from build123d import *

# Parameters (mm, degrees)
SKETCH_1_W          = 146
SKETCH_1_H          = 98
EXTRUDE_1_DEPTH     = 18
SKETCH_2_W          = 141
SKETCH_2_H          = 90
CUT_EXTRUDE_1_DEPTH = 14
SKETCH_3_W          = 91
SKETCH_3_H          = 90
CUT_EXTRUDE_2_DEPTH = 17
CUT_EXTRUDE_3_DEPTH = 17


with BuildPart() as part:
    # 草图1 → 凸台-拉伸1 (new body)
    with BuildSketch(Plane(origin=(0, 0, 0), x_dir=(1, 0, 0), z_dir=(0, 1, 0))):
        with Locations((-12.96875, -2.625)):
            Rectangle(SKETCH_1_W, SKETCH_1_H)
    extrude(amount=EXTRUDE_1_DEPTH)

    # 草图2 → 切除-拉伸1 (cut)
    with BuildSketch(Plane(origin=(0, 18, 0), x_dir=(1, 0, 0), z_dir=(0, 1, 0))):
        with Locations((-15.46875, -2.625)):
            Rectangle(SKETCH_2_W, SKETCH_2_H)
    extrude(amount=-CUT_EXTRUDE_1_DEPTH, mode=Mode.SUBTRACT)

    # 草图3 → 切除-拉伸2 (cut)
    with BuildSketch(Plane(origin=(0, 4, 0), x_dir=(1, 0, 0), z_dir=(0, 1, 0))):
        with Locations((9.53125, -2.625)):
            Rectangle(SKETCH_3_W, SKETCH_3_H)
    extrude(amount=-CUT_EXTRUDE_2_DEPTH, mode=Mode.SUBTRACT)

    # 草图5 → 切除-拉伸3 (cut)
    with BuildSketch(Plane(origin=(0, 4, 0), x_dir=(1, 0, 0), z_dir=(0, 1, 0))):
        with BuildLine():
            Line((-73.931388989, 24.875), (-77.931388989, 24.875))
            ThreePointArc((-77.931388989, 24.875), (-79.431388989, 26.375), (-77.931388989, 27.875))
            Line((-77.931388989, 27.875), (-73.931388989, 27.875))
            ThreePointArc((-73.931388989, 27.875), (-72.431388989, 26.375), (-73.931388989, 24.875))
        make_face()
        with BuildLine():
            Line((-73.931388989, 7.375), (-77.931388989, 7.375))
            ThreePointArc((-77.931388989, 7.375), (-79.431388989, 8.875), (-77.931388989, 10.375))
            Line((-77.931388989, 10.375), (-73.931388989, 10.375))
            ThreePointArc((-73.931388989, 10.375), (-72.431388989, 8.875), (-73.931388989, 7.375))
        make_face()
    extrude(amount=-CUT_EXTRUDE_3_DEPTH, mode=Mode.SUBTRACT)


solid = part.part
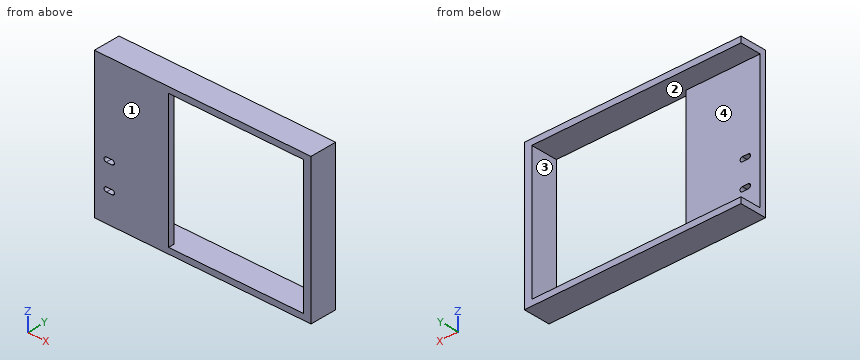
Input: part model. Units: mm. Frame: model coordinates. Face numbers are marked on the shaded views. A direction names the side the tool comes from. Give positions to 0.01 mm unless a question says otherwise; leave off trailing zeros. Write each loop counter-clockwise with the first axis right and the second up, starting at its lowest first coordinate (ties: lowest second). Pieces come first, ordered by that corner, then holes.
Q1. Section D-D, the plane x = -52. Output: boundary loops of the cut face in (y, z) (3 decimals), plus the area to 3 significant figures.
Q2. Material intervals for probe 1 along Z at (x, y) = (-60, 11.5) (3 decimals); probe 2 along X at (y, z) = (2.5, 43); probe 3 along X at (y, z) = (5.5, 30), sorted ascending.
Q3. Set-up query: the marked faces 1, 2, 3 and 4. Return all of +Z, -Z, +X, -X, +Y, -Y with unobstructed straight access to the full face (end or side cutting, diameter ignored); none if empty.
Q4. Section C-C, the plane y = 2. Output: boundary loops of the cut face in (x, z) (3 decimals), plus the area to 3 significant figures.
Q5. First-contact query: P1, Ø6, axis at x = -38.5, z = 30, coming from the +Y side. Flat tip, straight axial feed; report the tip coordinate or a pass-through.
Q6. Section B-B, the plane z = 0. Output: boundary loops of the cut face in (x, y), plus the area to 3 significant figures.
Q7. Section A-A, the plane x = -1. Output: boundary loops of the cut face in (y, z) (3 decimals), plus the area to 3 significant figures.
Filled in:
1. outline: (0, -46.375) - (18, -46.375) - (18, -42.375) - (4, -42.375) - (4, 47.625) - (18, 47.625) - (18, 51.625) - (0, 51.625) - close
1. area: 504 mm2
2. probe 1: z = -46.375 to -42.375, 47.625 to 51.625
2. probe 2: x = -85.97 to -35.97, 55.03 to 60.03
2. probe 3: x = 55.03 to 60.03
3. face 1: +Z, -Z, +X, -X, -Y
3. face 2: +Y
3. face 3: +Y, -Y
3. face 4: -X, +Y
4. outline: (-85.969, -46.375) - (60.031, -46.375) - (60.031, 51.625) - (-85.969, 51.625) - close; hole (-77.931, -27.875) - (-73.931, -27.875) arc R1.5 ccw to (-73.931, -24.875) - (-77.931, -24.875) arc R1.5 ccw to start; hole (-77.931, -10.375) - (-73.931, -10.375) arc R1.5 ccw to (-73.931, -7.375) - (-77.931, -7.375) arc R1.5 ccw to start; hole (-35.969, -42.375) - (55.031, -42.375) - (55.031, 47.625) - (-35.969, 47.625) - close
4. area: 6,080 mm2
5. P1: stops at y = 4
6. outline: (-85.97, 0) - (-35.97, 0) - (-35.97, 4) - (-85.97, 4) - close; (55.03, 0) - (60.03, 0) - (60.03, 18) - (55.03, 18) - close
6. area: 290 mm2
7. outline: (0, -46.375) - (18, -46.375) - (18, -42.375) - (0, -42.375) - close; (0, 47.625) - (18, 47.625) - (18, 51.625) - (0, 51.625) - close
7. area: 144 mm2
